from build123d import *

# Parameters (mm, degrees)
SKETCH1_R           = 1.25
SKETCH1_R_2         = 2
BOSS_EXTRUDE1_DEPTH = 1
SKETCH1_3_R         = 1.25
SKETCH1_3_R_2       = 2
BOSS_EXTRUDE2_DEPTH = 2
FILLET1_R           = 3


with BuildPart() as part:
    # Sketch1 → Boss-Extrude1 (new, symmetric)
    with BuildSketch(Plane.XY):
        with BuildLine():
            Line((-2.581223152, 3), (-2.581223152, -2))
            Line((-2.581223152, -2), (8, -2))
            Line((8, -2), (8, 9))
            Line((8, 9), (53, 9))
            Line((53, 9), (53, 14))
            ThreePointArc((53, 14), (50.1997341, 23.495673614), (42.695106585, 29.952443112))
            Line((42.695106585, 29.952443112), (5.569680923, 46.697301111))
            ThreePointArc((5.569680923, 46.697301111), (-2.260977773, 44.374109196), (-1.106198045, 36.288138625))
            ThreePointArc((-1.106198045, 36.288138625), (0.540780767, 33.340838667), (-0.061029462, 30.018649525))
            Line((-0.061029462, 30.018649525), (-12, 9.339745962))
            Line((-12, 9.339745962), (-12, 5.339745962))
            ThreePointArc((-12, 5.339745962), (-6.375794647, 7.852519152), (-2.581223152, 3))
        make_face()
        Circle(SKETCH1_R, mode=Mode.SUBTRACT)
        with Locations((0, 12.5)):
            Circle(SKETCH1_R_2, mode=Mode.SUBTRACT)
        with Locations((3, 41)):
            Circle(SKETCH1_R, mode=Mode.SUBTRACT)
    extrude(amount=BOSS_EXTRUDE1_DEPTH, both=True)

    # Sketch1_3 → Boss-Extrude2 (add, symmetric)
    with BuildSketch(Plane.XY):
        with BuildLine():
            Line((-2.581223152, -2), (8, -2))
            Line((8, -2), (8, 18))
            Line((8, 18), (-7, 18))
            Line((-7, 18), (-12, 9.339745962))
            Line((-12, 9.339745962), (-12, 5.339745962))
            ThreePointArc((-12, 5.339745962), (-6.375794647, 7.852519152), (-2.581223152, 3))
            Line((-2.581223152, 3), (-2.581223152, -2))
        make_face()
        Circle(SKETCH1_3_R, mode=Mode.SUBTRACT)
        with Locations((0, 12.5)):
            Circle(SKETCH1_3_R_2, mode=Mode.SUBTRACT)
    extrude(amount=BOSS_EXTRUDE2_DEPTH, both=True)

    # Fillet1
    fillet1_edges = [part.edges().sort_by_distance(p)[0] for p in [
        (-12, 9.339745962, 0),
        (8, 18, -1.5),
        (8, 18, 1.5),
    ]]
    fillet(fillet1_edges, radius=FILLET1_R)


solid = part.part
Geometry check sheet. Reference: the model listing, model coordinates, mm. A direction names the side the tool comes from. Give positions to 0.01 mm unless a question says otherwise; leave off trailing zeros. Write each loop counter-clockwise with the first axis right and the second up, starting at its lowest first coordinate (ties: lowest second). Pieces come first, ordered by that corner, then holes. Notation, with made-up numbers: (-29.5, -3) - (-3.5, -3) arc R18 cw to (-3.5, 22) - close; hole circle Ø10 at (-15.75, 59.25). An arc over 180 degrees is marked (long way). Put each result on its own line as item: value.
1. Thickness scan on line 1 (Y direction, x = 0, z = 0.25); line 2 (Y direction, x = 3, z = -0.3); line 3 (Z direction, x = 18, y = 38). Record the ranges inside material, lowest first.
Ans:
line 1: y = -2 to -1.25, 1.25 to 10.5, 14.5 to 30.13, 34.91 to 46.48
line 2: y = -2 to 39.75, 42.25 to 47.25
line 3: z = -1 to 1
2. Sectioned sample at D-D, the plane y = 41. Enter the section's corners in (x, z).
Ans:
outline: (-3.25, -1) - (1.75, -1) - (1.75, 1) - (-3.25, 1) - close; (4.25, -1) - (18.2, -1) - (18.2, 1) - (4.25, 1) - close
3. Sectioned sample at B-B, the plane y = 0. Enter the section's corners in (x, z), plus the area to 3 significant figures.
Ans:
outline: (-2.58, -2) - (-1.25, -2) - (-1.25, 2) - (-2.58, 2) - close; (1.25, -2) - (8, -2) - (8, 2) - (1.25, 2) - close
area: 32.3 mm²
4. Sectioned sample at C-C, the plane z = -0.2. Enter the section's corners in (x, y), plus the area to 3 significant figures.
Ans:
outline: (-12, 5.34) arc R5 cw to (-2.58, 3) - (-2.58, -2) - (8, -2) - (8, 9) - (53, 9) - (53, 14) arc R17.5 ccw to (42.7, 29.95) - (5.57, 46.7) arc R6.25 ccw to (-1.11, 36.29) arc R5 cw to (-0.06, 30.02) - (-11.6, 10.04) arc R3 ccw to (-12, 8.54) - close; hole circle Ø4 at (0, 12.5); hole circle Ø2.5 at (0, 0); hole circle Ø2.5 at (3, 41)
area: 1,730 mm²
5. Go/stop test with flat-tipped pins: pin 1 (1.5 mm diameter, centred on x = 0, y = 0, fed in from +Z); pin 2 (1 mm diameter, centred on x = 18.5, z = -0.5, fed in from +Y); pin 3 (3 mm diameter, centred on x = 3, y = 41, fed in from +Z); pin 4 (1 mm diameter, centred on y = 19, z = -0.5, fed in from +X). Record where each tip stops, or that it passes through.
Ans:
pin 1: passes through
pin 2: stops at y = 41.09
pin 3: stops at z = 1
pin 4: stops at x = 52.41
6. Sectioned sample at A-A, the plane x = 3. Enter the section's corners in (y, z).
Ans:
outline: (-2, -2) - (18, -2) - (18, -1) - (39.75, -1) - (39.75, 1) - (18, 1) - (18, 2) - (-2, 2) - close; (42.25, -1) - (47.25, -1) - (47.25, 1) - (42.25, 1) - close
7. Set-up check for faces 5 (the flat face through (23, 24, 1)), 6 (the flat face through (3, -2, 0)), 7 (the flat face through (23, 24, -1)): record each of +Z, -Z, +X, -X, +Y, -Y from which the full face is reachable in a straight line by a thin tool's end or side.
Ans:
face 5: +Z, +X, +Y
face 6: +Z, -Z, +X, -X, -Y
face 7: -Z, +X, +Y
8. Draft check along Y on faces 1 (the cylindrical face through (-11.9, 9.3, 0)), 2 (the flat face through (-2.581, 1, 0)), 3 (the cylindrical face through (-0.26, 14.483, -0.028)), 4 (the cylindrical face through (0.533, 33.388, 0.014)). Enter one of: +Y half, -Y half, draft (parallel to the pull), parting line (faces both ways), or undercut.
Ans:
face 1: +Y half
face 2: draft
face 3: undercut
face 4: undercut
